Geometry check sheet. Reference: the model listing, model coordinates, mm. Face numbers are marked on the shaded views. A direction names the side the tool comes from. Round coordinates to 2 decimals unless told otherwise and drop trailing zeros. Write each loop counter-clockwise with the first axis right and the second up, starting at its lowest first coordinate (ties: lowest second). Pieces come first, ordered by that corner, then holes. Notation, with made-up numbers: (49, 34) - (102, 34) arc R34 ccw to (102, 67) - close; hole circle Ø9 at (-17.5, -2.75). An arc over 180 degrees is marked (long way). Return JSON: item names as keys, results as strings.
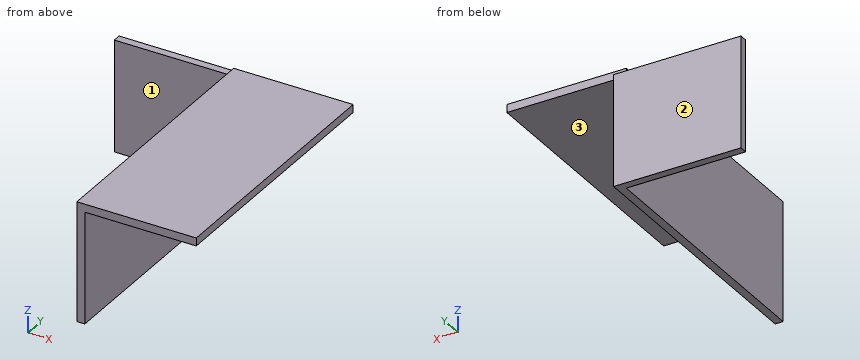
```python
from build123d import *

# Parameters (mm, degrees)
EXTRUDE_1_DEPTH     = 53
CUT_EXTRUDE_2_DEPTH = 20
SKETCH_6_W          = 14
SKETCH_6_H          = 1
EXTRUDE_2_DEPTH     = 16


with BuildPart() as part:
    # Эскиз1 → Бобышка-Вытянуть1 (new body)
    with BuildSketch(Plane(origin=(0, 0, 0), x_dir=(1, 0, 0), z_dir=(0, 1, 0))):
        Polygon((0, 0), (0, 15), (1, 15), (1, 1), (15, 1), (15, 0), align=None)
    extrude(amount=EXTRUDE_1_DEPTH)

    # Эскиз5 → Вырез-Вытянуть2 (cut)
    with BuildSketch(Plane(origin=(0, 53, 0), x_dir=(1, 0, 0), z_dir=(0, 1, 0))):
        Polygon((0, 0), (15, 0), (15, 1), (1, 1), (1, 15), (0, 15), align=None)
    extrude(amount=-CUT_EXTRUDE_2_DEPTH, mode=Mode.SUBTRACT)

    # Эскиз6 → Бобышка-Вытянуть2 (add)
    with BuildSketch(Plane(origin=(1, 0, 0), x_dir=(0, 0, -1), z_dir=(1, 0, 0))):
        with Locations((8, 33.5)):
            Rectangle(SKETCH_6_W, SKETCH_6_H)
    extrude(amount=-EXTRUDE_2_DEPTH)


solid = part.part
```
(1) Section check B-B, the plane y = 21. Enter the section's corners in (x, z), plus the area to 3 significant figures.
Response values:
{"outline": "(0, -15) - (1, -15) - (1, -1) - (15, -1) - (15, 0) - (0, 0) - close", "area": "29.0 mm^2"}
(2) Section check A-A, the plane z = -11. Enter the section's corners in (x, y), plus the area to 3 significant figures.
Response values:
{"outline": "(-15, 33) - (0, 33) - (0, 0) - (1, 0) - (1, 34) - (-15, 34) - close", "area": "49.0 mm^2"}
(3) Material ranges on line 1 along Z through (x, y) = (13.25, 25.5); line 2 along Y through (x, z) = (-1, -5.5); line 3 along X through (y, z) = (5, -13.25), recorded low to high. Write a range as [from, to].
Response values:
{"line 1": "z = [-1, 0]", "line 2": "y = [33, 34]", "line 3": "x = [0, 1]"}
(4) Gauge pin test, flat ends, axial feed: pin 1 (3 mm diameter, centred on y = 22.5, z = -8, fed in from -X); pin 2 (0.8 mm diameter, centred on x = 9, z = -0.5, fed in from +Y); pin 3 (3 mm diameter, centred on x = -4.5, z = -2.5, fed in from -Y); pin 4 (2 mm diameter, centred on x = -2, y = 16, fed in from -Z). Record the tip position at first contact, or that the pin passes through.
Response values:
{"pin 1": "stops at x = 0", "pin 2": "stops at y = 33", "pin 3": "stops at y = 33", "pin 4": "passes through"}
(5) Access from +Z, -Z, +X, -X, +Y, -Y to the whole of each face (thin tool, end or side, straight path). Record for the marked faces 1, 2 and 3.
Response values:
{"face 1": "+Z, -Z, -X, -Y", "face 2": "+Z, -Z, +X, -X, +Y", "face 3": "-Z, +X, +Y, -Y"}
(6) Section check C-C, the plane x = -3.25. Enter the section's corners in (y, z).
Response values:
{"outline": "(33, -15) - (34, -15) - (34, -1) - (33, -1) - close"}
(7) Section check D-D, the plane x = 5.75. Enter the section's corners in (y, z), plus the area to 3 significant figures.
Response values:
{"outline": "(0, -1) - (33, -1) - (33, 0) - (0, 0) - close", "area": "33.0 mm^2"}
